Read the model definition and answer for the solid it produces. Units are mm, in the model's axes. Face numbers are marked on the shaded views. A direction names the side the tool comes from. Give positions to 0.01 mm unless a question says otherwise; leave off trailing zeros. Order: outer loops, then holes, each group sorted by start corner. A loop starts at its lowest first (then second) coordinate and runs counter-clockwise, first axis right, second up. Notation, with made-up numbers: (21.25, 76) - (61.25, 76) arc R17 ccw to (61.25, 95) - close; hole circle Ø10 at (-22, 54.25). An arc over 180 degrees is marked (long way). Answer as CSV lines item,"result". Start each with the question number.
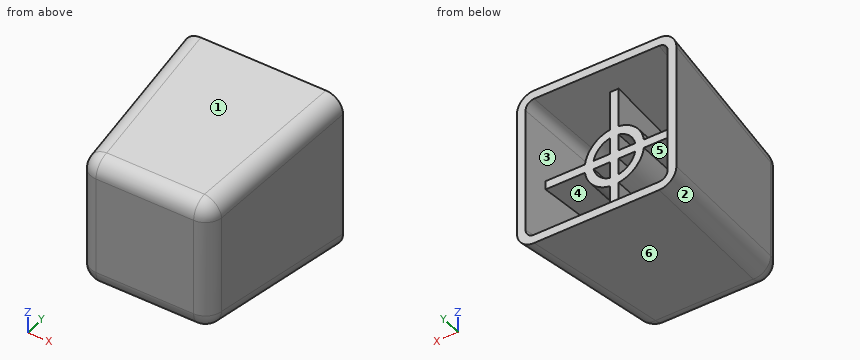
from build123d import *

# Parameters (mm, degrees)
SKETCH1_W          = 75
SKETCH1_H          = 75
BASE_EXTRUDE_DEPTH = 100
BASE_EXTRUDE_DRAFT = -5
FILLET1_R          = 10
SHELL1_T           = -5
RIB1_START         = -2.5
RIB1_DEPTH         = 5
RIB1_START_2       = -36.248793674
RIB1_2_OUTLINE_W   = 80
RIB1_2_OUTLINE_H   = 5
RIB1_2_DEPTH       = 72.497587348
RIB1_START_3       = 5
RIB1_3_DEPTH       = 80
RIB1_START_4       = 43.067212481
RIB1_4_OUTLINE_W   = 3.751206326
RIB1_4_OUTLINE_H   = 5
RIB1_4_DEPTH       = 41.932787519


with BuildPart() as part:
    # Sketch1 → Base-Extrude (with draft: the straight prism first)
    with BuildSketch(Plane(origin=(0, 0, 0), x_dir=(1, 0, 0), z_dir=(0, 1, 0))):
        Rectangle(SKETCH1_W, SKETCH1_H)
    extrude(amount=BASE_EXTRUDE_DEPTH)
    # Base-Extrude: the draft: its side faces are tilted about the plane it starts from
    base_extrude_sides = [part.faces().sort_by_distance(p)[0] for p in [
        (0, 50, -37.5),
        (-37.5, 50, 0),
        (0, 50, 37.5),
        (37.5, 50, 0),
    ]]
    draft(base_extrude_sides, Plane(origin=(0, 0, 0), x_dir=(1, 0, 0), z_dir=(0, 1, 0)), BASE_EXTRUDE_DRAFT)

    # Fillet1
    fillet1_edges = [part.edges().sort_by_distance(p)[0] for p in [
        (0, 0, 37.5),
        (-37.5, 0, 0),
        (0, 0, -37.5),
        (37.5, 0, 0),
        (41.874433176, 50, 41.874433176),
        (-41.874433176, 50, 41.874433176),
        (-41.874433176, 50, -41.874433176),
        (41.874433176, 50, -41.874433176),
    ]]
    fillet(fillet1_edges, radius=FILLET1_R)

    # Shell1
    shell1_openings = [part.faces().sort_by_distance(p)[0] for p in [
        (0, 100, 0),
    ]]
    offset(amount=SHELL1_T, openings=shell1_openings, kind=Kind.INTERSECTION)

    # Rib1: read off the stored shape, not the designer's step
    # Rib1 outline → Rib1 (add)
    with BuildSketch(Plane.YZ.offset(RIB1_START)):
        with BuildLine():
            Line((85, 39.917437212), (9.564221286, 33.31766175))
            ThreePointArc((9.564221286, 33.31766175), (6.313613316, 31.714639298), (5, 28.33668826))
            Line((5, 28.33668826), (5, -28.33668826))
            ThreePointArc((5, -28.33668826), (6.313613316, -31.714639298), (9.564221286, -33.31766175))
            Line((9.564221286, -33.31766175), (85, -39.917437212))
            Line((85, -39.917437212), (85, 39.917437212))
        make_face()
    extrude(amount=RIB1_DEPTH)

    # Rib1 2 outline → Rib1 2 (add)
    with BuildSketch(Plane.YZ.offset(RIB1_START_2)):
        with Locations((45, 0)):
            Rectangle(RIB1_2_OUTLINE_W, RIB1_2_OUTLINE_H)
    extrude(amount=RIB1_2_DEPTH)

    # Rib1 3 outline → Rib1 3 (add)
    with BuildSketch(Plane(origin=(0, 0, 0), x_dir=(1, 0, 0), z_dir=(0, 1, 0)).offset(RIB1_START_3)):
        with BuildLine():
            ThreePointArc((-2.5, -12.038877834), (-8.694382655, -8.694382655), (-12.038877834, -2.5))
            Line((-12.038877834, -2.5), (-17.11407953, -2.5))
            ThreePointArc((-17.11407953, -2.5), (-12.229916561, -12.229916561), (-2.5, -17.11407953))
            Line((-2.5, -17.11407953), (-2.5, -12.038877834))
        make_face()
        with BuildLine():
            ThreePointArc((2.5, -17.11407953), (12.229916561, -12.229916561), (17.11407953, -2.5))
            Line((17.11407953, -2.5), (12.038877834, -2.5))
            ThreePointArc((12.038877834, -2.5), (8.694382655, -8.694382655), (2.5, -12.038877834))
            Line((2.5, -12.038877834), (2.5, -17.11407953))
        make_face()
        with BuildLine():
            Line((-17.11407953, 2.5), (-12.038877834, 2.5))
            ThreePointArc((-12.038877834, 2.5), (-8.694382655, 8.694382655), (-2.5, 12.038877834))
            Line((-2.5, 12.038877834), (-2.5, 17.11407953))
            ThreePointArc((-2.5, 17.11407953), (-12.229916561, 12.229916561), (-17.11407953, 2.5))
        make_face()
        with BuildLine():
            ThreePointArc((17.11407953, 2.5), (12.229916561, 12.229916561), (2.5, 17.11407953))
            Line((2.5, 17.11407953), (2.5, 12.038877834))
            ThreePointArc((2.5, 12.038877834), (8.694382655, 8.694382655), (12.038877834, 2.5))
            Line((12.038877834, 2.5), (17.11407953, 2.5))
        make_face()
    extrude(amount=RIB1_3_DEPTH)

    # Rib1 4 outline → Rib1 4 (add)
    with BuildSketch(Plane(origin=(0, 0, 0), x_dir=(1, 0, 0), z_dir=(0, 1, 0)).offset(RIB1_START_4)):
        with Locations((-38.124396837, 0)):
            Rectangle(RIB1_4_OUTLINE_W, RIB1_4_OUTLINE_H)
        with Locations((38.124396837, 0)):
            Rectangle(RIB1_4_OUTLINE_W, RIB1_4_OUTLINE_H)
    extrude(amount=RIB1_4_DEPTH)


solid = part.part
(1) Section D-D, the plane x = 8 is taken. Write down the section's boundary in (y, z).
(2) Section A-A, the plane z = 26.5 is taken. Write down the section's boundary in (x, y), and give its area (3 significant figures).
(3) Flat-ended cylindrical pins translate along their axes: pin 1 Ø3 at (y, z) = (36.5, 32.5) entering from +X; pin 2 Ø10.5 at (y, z) = (40.5, 8) entering from +X; pin 3 Ø11.5 at (y, z) = (55.5, -23) entering from -X. Find the tip coordinate at first contact, or state that the pin passes through.
(4) Determine the mould class of the marked faces 1, 2, 3 and 4 for opening direction X: released by +X, released by -X, zero draft, split by the parting line, or undercut.
(5) Section B-B, the plane x = 25 is taken. Write down the section's boundary in (y, z).
(6) Straight lines are drawn through the part: line 1 (Z direction, x = 35, y = 43.5); line 2 (Z direction, x = -25.5, y = 12); line 3 (X direction, y = 16.5, z = -32). For each, find the intervals that lie inside material, in ascending order. Write a range as [from, to].
(7) Section C-C, the plane y = 66 is taken. State how many separate pieces and enclosed holes the cut face has, and give its area (3 significant figures).
(8) Which of the six approach directions +Z, -Z, +X, -X, +Y, -Y give full straight-line access (tool end or side, diameter ignored) to the marked faces 5 and 6?
Checks:
1,outline,"(0, -28.34) arc R10 ccw to (9.13, -38.3) - (100, -46.25) - (100, -41.23) - (9.56, -33.32) arc R5 cw to (5, -28.34) - (5, -15.33) - (85, -15.33) - (85, -9.34) - (5, -9.34) - (5, -2.5) - (85, -2.5) - (85, 2.5) - (5, 2.5) - (5, 9.34) - (85, 9.34) - (85, 15.33) - (5, 15.33) - (5, 28.34) arc R5 cw to (9.56, 33.32) - (100, 41.23) - (100, 46.25) - (9.13, 38.3) arc R10 ccw to (0, 28.34) - close"
2,outline,"(-46.25, 100) - (-38.3, 9.13) arc R10 ccw to (-28.34, 0) - (28.34, 0) arc R10 ccw to (38.3, 9.13) - (46.25, 100) - (41.23, 100) - (33.32, 9.56) arc R5 cw to (28.34, 5) - (2.5, 5) - (2.5, 85) - (-2.5, 85) - (-2.5, 5) - (-28.34, 5) arc R5 cw to (-33.32, 9.56) - (-41.23, 100) - close"
2,area,"1,700 mm²"
3,pin 1,"stops at x = 40.77"
3,pin 2,"stops at x = 41.5"
3,pin 3,"stops at x = -42.86"
4,face 1,"zero draft"
4,face 2,"released by -X"
4,face 3,"undercut"
4,face 4,"undercut"
5,outline,"(0, -28.34) arc R10 ccw to (9.13, -38.3) - (100, -46.25) - (100, -41.23) - (9.56, -33.32) arc R5 cw to (5, -28.34) - (5, -2.5) - (85, -2.5) - (85, 2.5) - (5, 2.5) - (5, 28.34) arc R5 cw to (9.56, 33.32) - (100, 41.23) - (100, 46.25) - (9.13, 38.3) arc R10 ccw to (0, 28.34) - close"
6,line 1,"z = [-40.61, -34.65], [-2.5, 2.5], [34.65, 40.61]"
6,line 2,"z = [-38.55, -33.53], [-2.5, 2.5], [33.53, 38.55]"
6,line 3,"x = [-38.48, -32.88], [-2.5, 2.5], [32.88, 38.48]"
7,separate pieces,"1"
7,enclosed holes,"8"
7,area,"2,680 mm²"
8,face 5,"+Y"
8,face 6,"-Z, +X, -X, -Y"
